Autodesk Inventor part; units mm, degrees
ref_plane "YZ Plane" through (0, 0, 0) normal (1, 0, 0) x (0, 1, 0)
ref_plane "XZ Plane" through (0, 0, 0) normal (0, 1, 0) x (-1, 0, 0)
ref_plane "XY Plane" through (0, 0, 0) normal (0, 0, 1) x (1, 0, 0)
sketch "Boceto1" plane through (0, 0, 0) normal (0, 0, 1) x (1, 0, 0)
  line L0 (-4.78, 4.78) -> (4.78, 4.78)
  line L1 (4.78, 4.78) -> (4.78, -4.78)
  line L2 (4.78, -4.78) -> (-4.78, -4.78)
  line L3 (-4.78, -4.78) -> (-4.78, 4.78)
  line L4 (-4.78, 4.78) -> (4.78, -4.78) construction
  line L5 (4.78, 4.78) -> (-4.78, -4.78) construction
  point P0 (0, 0)
  dimension "d0" = 9.56
  dimension "d1" = 9.56
extrude "Extrusión1" add sketch "Boceto1" along normal mid plane 4.6
sketch "Boceto2" plane through (0, 0, 2.3) normal (0, 0, 1) x (1, 0, 0)
  line L0 (-4.78, 4.78) -> (-3.58, 4.78)
  line L1 (-3.58, 4.78) -> (-3.58, 3.92)
  line L2 (-3.58, 3.92) -> (-4.78, 3.92)
  line L3 (-4.78, 3.92) -> (-4.78, 4.78)
  point P0 (0, 0)
  dimension "d4" = 1.2
  dimension "d5" = 0.86
extrude "Extrusión2" add sketch "Boceto2" along normal blind 0.37
mirror "Simetría1" about plane through (0, 0, 0) normal (0, 1, 0) of "Extrusión2"
mirror "Simetría2" about plane through (0, 0, 0) normal (1, 0, 0) of "Extrusión2", "Simetría1"
sketch "Boceto5" plane through (0, 0, 2.3) normal (0, 0, 1) x (1, 0, 0)
  line L0 (-3.58, 3.92) -> (-4.78, 3.92)
  line L1 (-4.78, -3.92) -> (-4.41, -3.92)
  line L2 (-4.41, -3.92) -> (-4.41, 3.92)
  line L3 (-4.41, 3.92) -> (-4.78, 3.92)
  line L4 (-4.78, 3.92) -> (-4.78, -3.92)
  point P0 (0, 0)
  dimension "d21" = 0.37
extrude "Extrusión4" cut sketch "Boceto5" against normal through all
sketch "Boceto6" plane through (0, 0, 2.3) normal (0, 0, 1) x (1, 0, 0)
  line L0 (-4.41, 3.92) -> (-4.41, -3.92)
  line L1 (-4.41, -3.92) -> (-3.58, -3.92)
  line L2 (-3.58, -2.85) -> (-3.58, -1.99)
  line L3 (-3.58, -1.99) -> (-4.41, -1.99)
  line L4 (-4.41, -2.85) -> (-3.58, -2.85)
  line L5 (-3.58, -4.78) -> (-4.78, -4.78)
  point P0 (0, 0)
  dimension "d24" = 1.93
  dimension "d25" = 0.86
  dimension "d26" = 0.86
extrude "Extrusión5" cut sketch "Boceto6" against normal through all
mirror "Simetría3" about plane through (0, 0, 0) normal (0, 1, 0) of "Extrusión5"
sketch "Boceto7" plane through (0, 0, 2.3) normal (0, 0, 1) x (1, 0, 0)
  line L0 (-3.58, 1.99) -> (-4.41, 1.99)
  line L1 (-4.41, 1.99) -> (-4.41, -1.99)
  line L2 (-4.41, -1.99) -> (-3.58, -1.99)
  line L3 (-3.58, -2.85) -> (-4.41, -2.85)
  line L4 (-3.58, 2.85) -> (-3.58, 1.99)
  line L5 (-4.41, -0.43) -> (-3.58, -0.43)
  line L6 (-3.58, -0.43) -> (-3.58, 0.43)
  line L7 (-3.58, 0.43) -> (-4.41, 0.43)
  point P0 (0, 0)
  dimension "d29" = 3.98
  dimension "d30" = 0.86
  dimension "d31" = 0.86
  dimension "d32" = 1.56
  dimension "d33" = 1.56
extrude "Extrusión6" cut sketch "Boceto7" against normal through all
sketch "Boceto8" plane through (0, 0, -2.3) normal (0, 0, -1) x (-1, 0, 0)
  circle A0 centre (0, 0) radius 0.5
  dimension "d36" = 1
hole "Hole1" at (0, 0, -2.3) direction (0, 0, 1) diameter 1 depth 2
sketch "Boceto9" plane through (0, 0, 2.3) normal (0, 0, 1) x (1, 0, 0)
  circle A0 centre (0, -2.42) radius 0.25
  circle A1 centre (0, 0) radius 0.25
  circle A2 centre (0, 2.42) radius 0.25
  dimension "d44" = 0.5
  dimension "d45" = 0.5
  dimension "d47" = 0.5
extrude "Extrusión7" add sketch "Boceto9" along normal blind 6.5
properties part number "BasePotenciometro"
Check sheet for the modelled part. Datum: model origin and axes. Units: mm. A direction names the side the tool comes from. Give positions to 0.01 mm unless a question says otherwise; leave off trailing zeros. Order: outer loops, then holes, each group sorted by start corner. A loop starts at its lowest first (then second) coordinate and runs counter-clockwise, first axis right, second up. Notation, with made-up numbers: (26.25, 33) -> (71.25, 33) arc R9 ccw to (71.25, 47) -> close; hole circle Ø1 at (49.5, 53.5). An arc over 180 degrees is marked (long way). Use CSV: the item, a comma, the result in double quotes. Start each with the question number.
1) Sectioned sample at D-D, the plane y = 4.25. Record the boundary of the cut face in (x, z).
2) Mould release check, pull along Y, two halves, no side actions. Record for faces 1 (the face through (-4, -2.85, 0)), 2 (the face through (4.2, 4.4, 2.67)), 3 (the face through (0, -4.78, 0)): released by +Y, released by -Y, zero draft, split by the parting line, or undercut.
3) Sectioned sample at B-B, the plane z = 4.5. Record the boundary of the cut face in (x, y).
4) Sectioned sample at C-C, the plane x = 1. Record the boundary of the cut face in (y, z), plus the area to 3 significant figures.
5) Set-up check for faces 4 (the face through (-4.2, 4.4, 2.67)), 5 (the face through (-4, 0.43, 0)): record each of +Z, -Z, +X, -X, +Y, -Y from which the full face is reachable in a straight line by a thin tool's end or side.
6) Sectioned sample at A-A, the plane y = -2.42. Record the boundary of the cut face in (x, z), plus the area to 3 significant figures.
7) Material ranges on line 1 (X direction, y = 0, z = -1.25); line 2 (Y direction, x = 0, z = -1.35); line 3 (X direction, y = 1, z = 0.75), recorded low to high. Write a range as from..to.
8) Go/stop test with flat-tipped pins: P1, Ø3, axis at x = -3.5, y = -2.5, coming from the +Z side; P2, Ø1.5, axis at x = 1.5, y = 2.5, coming from the +Z side; P3, Ø0.5, axis at y = 1, z = -1, coming from the -X side. Record where each tip stops, or that it passes through.
Recorded:
1,outline,"(-4.78, -2.3) -> (4.78, -2.3) -> (4.78, 2.67) -> (3.58, 2.67) -> (3.58, 2.3) -> (-3.58, 2.3) -> (-3.58, 2.67) -> (-4.78, 2.67) -> close"
2,face 1,"undercut"
2,face 2,"zero draft"
2,face 3,"released by -Y"
3,outline,"circle Ø0.5 at (0, -2.42); circle Ø0.5 at (0, 0); circle Ø0.5 at (0, 2.42)"
4,outline,"(-4.78, -2.3) -> (4.78, -2.3) -> (4.78, 2.3) -> (-4.78, 2.3) -> close"
4,area,"44.0 mm2"
5,face 4,"+Z, +X, -X, +Y, -Y"
5,face 5,"+Z, -Z, -X"
6,outline,"(-3.58, -2.3) -> (4.78, -2.3) -> (4.78, 2.3) -> (0.25, 2.3) -> (0.25, 8.8) -> (-0.25, 8.8) -> (-0.25, 2.3) -> (-3.58, 2.3) -> close"
6,area,"41.7 mm2"
7,line 1,"-3.58..-0.5, 0.5..4.78"
7,line 2,"-4.78..-0.5, 0.5..4.78"
7,line 3,"-4.41..4.78"
8,P1,"z = 2.67"
8,P2,"z = 2.3"
8,P3,"x = -4.41"
